from build123d import *

# Parameters (mm, degrees)
F0_W     = 23.200736
F0_H     = 11.930093
F1_DEPTH = 10.16
F2_T     = -2.54
F4_D     = 1.524


with BuildPart() as f1:
    # F0 (on Front) → F1 (new body)
    with BuildSketch(Plane.XZ):
        with Locations((-46.540994, 30.285004)):
            Rectangle(F0_W, F0_H)
    extrude(amount=F1_DEPTH)

    # F2
    f2_openings = [f1.faces().sort_by_distance(p)[0] for p in [
        (-46.540994, -5.08, 36.250051),
        (-58.141362, -5.08, 30.285005),
        (-34.940626, -5.08, 30.285005),
    ]]
    offset(amount=F2_T, openings=f2_openings)

    # F4 (through all)
    with Locations(Plane(origin=(0, 0, 0), x_dir=(-1, 0, 0), z_dir=(0, 1, 0))):
        with Locations((37.589088, 30.788029), (53.718481, 30.440666)):
            Hole(F4_D / 2)


solid = f1.part
Read the model definition and answer for the solid it produces. Units are mm, in the model's axes. A direction names the side the tool comes from. Round coordinates to 2 decimals unless told otherwise and drop trailing zeros. Write each loop counter-clockwise with the first axis right and the second up, starting at its lowest first coordinate (ties: lowest second). Pieces come first, ordered by that corner, then holes.
1. Straight lines are drawn through the part: L1, parallel to Y at x = -50.75, z = 31.25; L2, parallel to Z at x = -48, y = -5.5; L3, parallel to Z at x = -37.75, y = -8. For each, find the intervals that lie inside material, in ascending order.
2. The part is cut by section B-B, the plane x = -47.5. Determine the outline of the cut face in (y, z).
3. The part is cut by section A-A, the plane z = 27.25. Determine the outline of the cut face in (x, y).
4. Which of the six approach directions +Z, -Z, +X, -X, +Y, -Y give full straight-line access (tool end or side, diameter ignored) to faces 4 (the face through (-47, -2.54, 32)), 5 (the face through (-47, -5, 24.32))?
5. The part is cut by section C-C, the plane y = -3.25. Determine the outline of the cut face in (x, z), then the cut area to 3 significant figures.
6. Given pin 1 Ø2.5 at (x, y) = (-44, -5) entering from +Z; pin 2 Ø2.5 at (x, z) = (-53.72, 30.44) entering from +Y, each flat-ended and moving along its own axis, determine where each tip first touches the part or whether it passes through.
7. Determine the mould class of faces 1 (the face through (-38.19, -8.91, 30.32)), 2 (the face through (-58.141, -5, 26)), 3 (the face through (-47, -5, 26.86)) for opening direction X: pulls with the +X half, pulls with the -X half, needs draft (parallel to the pull), parting line crosses it, or undercut.
Values:
1. L1: y = -10.16 to -7.62, -2.54 to 0
1. L2: z = 24.32 to 26.86
1. L3: z = 24.32 to 30.04, 31.53 to 36.25
2. outline: (-10.16, 24.32) - (0, 24.32) - (0, 36.25) - (-2.54, 36.25) - (-2.54, 26.86) - (-7.62, 26.86) - (-7.62, 36.25) - (-10.16, 36.25) - close
3. outline: (-58.14, -10.16) - (-34.94, -10.16) - (-34.94, -7.62) - (-58.14, -7.62) - close; (-58.14, -2.54) - (-34.94, -2.54) - (-34.94, 0) - (-58.14, 0) - close
4. face 4: +Z, +X, -X
4. face 5: -Z, +X, -X, +Y, -Y
5. outline: (-58.14, 24.32) - (-34.94, 24.32) - (-34.94, 26.86) - (-58.14, 26.86) - close
5. area: 58.9 mm2
6. pin 1: stops at z = 26.86
6. pin 2: stops at y = 0
7. face 1: undercut
7. face 2: pulls with the -X half
7. face 3: needs draft
